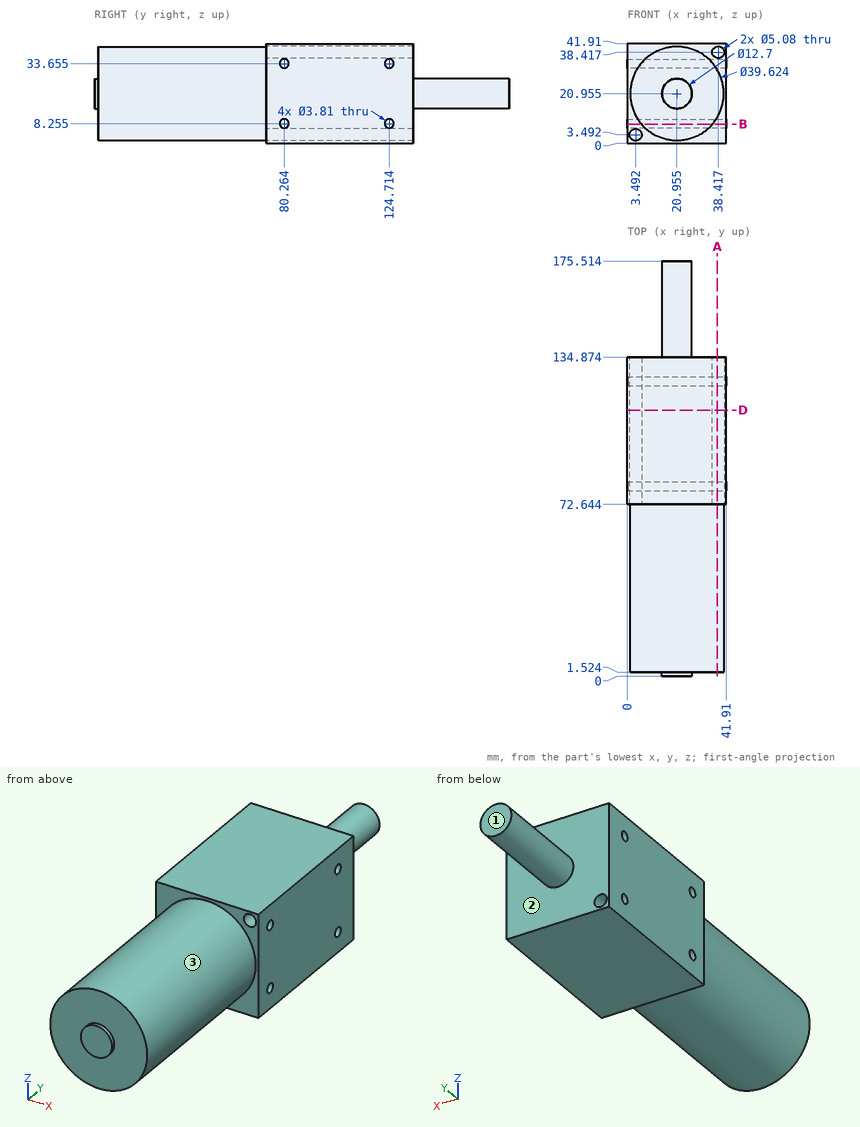
Design review of the part shown in the three views and the two pictorial views. Dimensions are in mm from the part's minimum x, y and z. A direction names the side the tool comes from. Give positions to 0.01 mm unless a question says otherwise; leave off trailing zeros. Write each loop counter-clockwise with the first axis right and the second up, starting at its lowest first coordinate (ties: lowest second). Pieces come first, ordered by that corner, then holes. Notation, with made-up numbers: M 29,34 L 53,34 A6 ccw 53,39 Z; hole C -2,30.5 d9. An arc over 180 degrees is marked long. One line per question, with ' | ' between items. Start each with the question number.
Item 1: For the marked faces 1, 2 and 3, list the 3-axis set-ups (+Z, -Z, +X, -X, +Y, -Y) from which the entire face can be reached by the end or side of a thin tool; tool diameter is ignored.
Item 2: For pin 1 (6 mm diameter, centred on x = 13, y = 46, fed in from -Z); pin 2 (6 mm diameter, centred on x = 38.42, z = 38.42, fed in from +Y); pin 3 (1 mm diameter, centred on y = 71, z = 15.5, fed in from +X), all flat-tipped, find the tip position at first contact; note any pin that passes through.
Item 3: We need section B-B on z = 8. Write out the cut boundary in (x, y) (1 decimal).
Item 4: Wall thickness on line 1 (Y direction, x = 22.5, z = 34) (1 decimal); line 2 (Y direction, x = 7.5, z = 9) (1 decimal); line 3 (Y direction, x = 12.5, z = 19) (1 decimal): over which ranges is each line inside the solid? List them lowest first. Write a range as from..to.
Item 5: We need section D-D on y = 112.5. Write out the cut boundary in (x, z), plus the area to 3 significant figures.
Item 6: We need section A-A on x = 38. Give the number of separate pieces and of enclosed holes in the cut face, plus the area to 3 significant figures.
Results found:
1) face 1: +Z, -Z, +X, -X, +Y | face 2: +Y | face 3: -Y
2) pin 1: stops at z = 1.77 | pin 2: stops at y = 134.87 | pin 3: stops at x = 40.14
3) outline: M 0,72.6 L 6,72.6 L 6,1.5 L 35.9,1.5 L 35.9,72.6 L 41.9,72.6 L 41.9,78.4 L 0,78.4 Z; M 0,82.2 L 41.9,82.2 L 41.9,122.8 L 0,122.8 Z; M 0,126.6 L 41.9,126.6 L 41.9,134.9 L 0,134.9 Z
4) line 1: y = 1.5..78.4, 82.1..122.8, 126.6..134.9 | line 2: y = 1.5..78.5, 82..123, 126.5..134.9 | line 3: y = 1.5..134.9
5) outline: M 0,0 L 41.91,0 L 41.91,41.91 L 0,41.91 Z; hole C 3.49,3.49 d5.08; hole C 38.42,38.42 d5.08 | area: 1,720 mm2
6) separate pieces: 2 | enclosed holes: 4 | area: 3,690 mm2
